Geometry: final body of the model. Coordinates: model frame, mm. A direction names the side the tool comes from. Round coordinates to 2 decimals unless told otherwise and drop trailing zeros. Write each loop counter-clockwise with the first axis right and the second up, starting at its lowest first coordinate (ties: lowest second). Pieces come first, ordered by that corner, then holes. Notation, with made-up numbers: M 32,4.25 L 55,4.25 A16 ccw 55,29.25 Z; hole C -9.5,78.25 d4. An arc over 180 degrees is marked long. Put each result on its own line as item: value. Start each with the question number.
```python
from build123d import *

# Parameters (mm, degrees)
EXTRUDE_1_DEPTH        = 5
SKETCH_2_R             = 14
SKETCH_2_R_2           = 12.3
EXTRUDE_2_DEPTH        = 4.5
SKETCH_3_W             = 14.3
SKETCH_3_H             = 14.3
EXTRUDE_3_DEPTH        = 3
SKETCH_4_R             = 3.6
CUT_EXTRUDE_2_DEPTH    = 24.286262044
HOLE_WIZARD_M2_1_D     = 2.4
HOLE_WIZARD_M2_1_DEPTH = 3
HOLE_WIZARD_M2_1_TIP   = 0.721032743


with BuildPart() as part:
    # 스케치1 → 보스-돌출1 (new body)
    with BuildSketch(Plane.XY):
        with BuildLine():
            Line((-6, 16), (6, 16))
            ThreePointArc((6, 16), (11.656854249, 13.656854249), (14, 8))
            Line((14, 8), (14, -8))
            ThreePointArc((14, -8), (11.656854249, -13.656854249), (6, -16))
            Line((6, -16), (-6, -16))
            ThreePointArc((-6, -16), (-11.656854249, -13.656854249), (-14, -8))
            Line((-14, -8), (-14, 8))
            ThreePointArc((-14, 8), (-11.656854249, 13.656854249), (-6, 16))
        make_face()
    extrude(amount=EXTRUDE_1_DEPTH)

    # 스케치2 → 보스-돌출2 (add)
    with BuildSketch(Plane.XY.offset(5)):
        Circle(SKETCH_2_R)
        Circle(SKETCH_2_R_2, mode=Mode.SUBTRACT)
    extrude(amount=EXTRUDE_2_DEPTH)

    # 스케치3 → 보스-돌출3 (add)
    with BuildSketch(Plane(origin=(0, 0, 0), x_dir=(-1, 0, 0), z_dir=(0, 0, -1))):
        with BuildLine():
            Line((-7.9, 7.9), (-3.3, 7.9))
            Line((-3.3, 7.9), (-3.3, 8.6))
            Line((-3.3, 8.6), (-6, 8.6))
            Line((-6, 8.6), (-6, 9.8))
            Line((-6, 9.8), (-7.3, 9.8))
            Line((-7.3, 9.8), (-7.3, 14.8))
            Line((-7.3, 14.8), (-6, 14.8))
            Line((-6, 14.8), (-6, 16))
            Line((-6, 16), (6, 16))
            Line((6, 16), (6, 14.8))
            Line((6, 14.8), (7.3, 14.8))
            Line((7.3, 14.8), (7.3, 9.8))
            Line((7.3, 9.8), (6, 9.8))
            Line((6, 9.8), (6, 8.6))
            Line((6, 8.6), (2.9, 8.6))
            Line((2.9, 8.6), (2.9, 7.9))
            Line((2.9, 7.9), (7.9, 7.9))
            Line((7.9, 7.9), (7.9, 2.4))
            Line((7.9, 2.4), (10, 2.4))
            ThreePointArc((10, 2.4), (12.4, 0), (10, -2.4))
            Line((10, -2.4), (7.9, -2.4))
            Line((7.9, -2.4), (7.9, -7.9))
            Line((7.9, -7.9), (-7.9, -7.9))
            Line((-7.9, -7.9), (-7.9, -2.4))
            Line((-7.9, -2.4), (-10, -2.4))
            ThreePointArc((-10, -2.4), (-12.4, 0), (-10, 2.4))
            Line((-10, 2.4), (-7.9, 2.4))
            Line((-7.9, 2.4), (-7.9, 7.9))
        make_face()
        Rectangle(SKETCH_3_W, SKETCH_3_H, mode=Mode.SUBTRACT)
    extrude(amount=EXTRUDE_3_DEPTH)

    # 스케치4 → 컷-돌출2 (cut, through all)
    with BuildSketch(Plane.XY):
        Circle(SKETCH_4_R)
    extrude(amount=CUT_EXTRUDE_2_DEPTH, mode=Mode.SUBTRACT)

    # M2 여유 구멍1
    with Locations(Plane(origin=(-10, 0, -3), x_dir=(-1, 0, 0), z_dir=(0, 0, -1))):
        with Locations((0, 0), (-20, 0)):
            Hole(HOLE_WIZARD_M2_1_D / 2, depth=HOLE_WIZARD_M2_1_DEPTH)
            with Locations((0, 0, -(HOLE_WIZARD_M2_1_DEPTH + HOLE_WIZARD_M2_1_TIP / 2))):  # 118° drill point
                Cone(0, HOLE_WIZARD_M2_1_D / 2, HOLE_WIZARD_M2_1_TIP, mode=Mode.SUBTRACT)


solid = part.part
```
1) Draft query along Y for faces 6 (the face through (-1, -14.5, 5)), 7 (the face through (-11.719, 13.594, 2.465)), 8 (the face through (5, 8.6, -1)), 9 (the face through (3, 3, 0)). Return one class per face: +Y half, -Y half, draft (parallel to the pull), parting line (faces both ways), or undercut.
2) Section A-A, the plane x = 0. Output: boundary loops of the cut face in (y, z).
3) Ray query, probe 1 along X at (y, z) = (0, -1.3); probe 2 along Y at (x, z) = (2.25, -1); probe 3 along Y at (x, z) = (-10, -1.75). Return the intervals inside material, ascending.
4) First-contact query: pin 1 (1 mm diameter, centred on x = -7, z = -2, fed in from -Y); pin 2 (5 mm diameter, centred on x = 11, y = -4, fed in from +Z); pin 3 (1 mm diameter, centred on x = -9, z = 3.5, fed in from -Y); pin 4 (3 mm diameter, centred on x = -10, y = 0, fed in from +Z). Flat tips, straight axial feed; report the tip coordinate or a pass-through.
5) Section B-B, the plane z = 3.25. Output: boundary loops of the cut face in (x, y), and give its area (3 significant figures).
6) Access query for faces 1 (the face through (-4, 8.6, -1)), 2 (the face through (-7.9, -5, -1)), 3 (the face through (7.9, 5, -1)), 4 (the face through (12.4, -0.05, -1.48)), 5 (the face through (-3, -3, 5)). Directions: +Z, -Z, +X, -X, +Y, -Y. A direction counts if a zero-diameter tool reaches every point of the face in a straight line with its end or side. Return the directions, or none.
7) Section D-D, the plane y = 9. Output: boundary loops of the cut face in (x, z), and give its area (3 significant figures).
8) Section C-C, the plane y = -2. Output: boundary loops of the cut face in (x, z), and give its area (3 significant figures).
Solved:
1. face 6: draft
1. face 7: +Y half
1. face 8: undercut
1. face 9: undercut
2. outline: M -16,0 L -7.9,0 L -7.9,-3 L -7.15,-3 L -7.15,0 L -3.6,0 L -3.6,5 L -12.3,5 L -12.3,9.5 L -14,9.5 L -14,5 L -16,5 Z; M 3.6,0 L 7.15,0 L 7.15,-3 L 16,-3 L 16,5 L 14,5 L 14,9.5 L 12.3,9.5 L 12.3,5 L 3.6,5 Z
3. probe 1: x = -12.4 to -11.2, -8.8 to -7.15, 7.15 to 8.8, 11.2 to 12.4
3. probe 2: y = -7.9 to -7.15, 7.15 to 16
3. probe 3: y = -2.4 to -1.2, 1.2 to 2.4
4. pin 1: stops at y = -7.9
4. pin 2: stops at z = 9.5
4. pin 3: stops at y = -15.6
4. pin 4: stops at z = 5
5. outline: M -14,-8 A8 ccw -6,-16 L 6,-16 A8 ccw 14,-8 L 14,8 A8 ccw 6,16 L -6,16 A8 ccw -14,8 Z; hole C 0,0 d7.2
5. area: 800 mm2
6. face 1: -Z, -X
6. face 2: -Z, -X, -Y
6. face 3: -Z, +X, +Y
6. face 4: -Z, +X
6. face 5: +Z
7. outline: M -13.94,0 L -6,0 L -6,-3 L 6,-3 L 6,0 L 13.94,0 L 13.94,5 L 10.72,5 L 10.72,9.5 L 8.38,9.5 L 8.38,5 L -8.38,5 L -8.38,9.5 L -10.72,9.5 L -10.72,5 L -13.94,5 Z
7. area: 196 mm2
8. outline: M -14,0 L -11.33,0 L -11.33,-3 L -7.15,-3 L -7.15,0 L -2.99,0 L -2.99,5 L -12.14,5 L -12.14,9.5 L -13.86,9.5 L -13.86,5 L -14,5 Z; M 2.99,0 L 7.15,0 L 7.15,-3 L 11.33,-3 L 11.33,0 L 14,0 L 14,5 L 13.86,5 L 13.86,9.5 L 12.14,9.5 L 12.14,5 L 2.99,5 Z
8. area: 151 mm2
